```python
from build123d import *

# Parameters (mm, degrees)
F0_W     = 80
F0_H     = 80
F1_DEPTH = 80
F2_R     = 17.5
F3_DEPTH = 25
F4_R     = 17.5
F5_DEPTH = 80.001
F6_T     = -2.5


with BuildPart() as f1:
    # F0 (on Front) → F1 (new body)
    with BuildSketch(Plane.XZ):
        Rectangle(F0_W, F0_H)
    extrude(amount=F1_DEPTH)

    # F2 (on face) → F3 (join)
    with BuildSketch(Plane.XZ.offset(80)):
        Circle(F2_R)
    extrude(amount=F3_DEPTH)

    # F4 (on face) → F5 (cut, through all)
    with BuildSketch(Plane.XY.offset(40)):
        with Locations((0, -40)):
            Circle(F4_R)
    extrude(amount=-F5_DEPTH, mode=Mode.SUBTRACT)

    # F6
    f6_openings = [f1.faces().sort_by_distance(p)[0] for p in [
        (-38.868629, -40, -40),
    ]]
    offset(amount=F6_T, openings=f6_openings, kind=Kind.INTERSECTION)


solid = f1.part
```
Design review of the part built by this model. Coordinates are the model's own, in mm. A direction names the side the tool comes from. Give positions to 0.01 mm unless a question says otherwise; leave off trailing zeros. Order: outer loops, then holes, each group sorted by start corner. A loop starts at its lowest first (then second) coordinate and runs counter-clockwise, first axis right, second up. Notation, with made-up numbers: M 8.25,74.5 L 60.25,74.5 A14 ccw 60.25,82.5 Z; hole C 19.25,43.5 d11. An arc over 180 degrees is marked long. One line per question, with ' | ' between items. Start each with the question number.
Q1. For L1, parallel to Y at x = 0, z = -7; L2, parallel to Y at x = 0, z = 18.5; L3, parallel to Y at x = 35, z = 34.5, list the stretches that pass through material, from the lowest coordinate up. Write a range as [from, to].
Q2. Machinability: for faces 5 (the face through (-37.5, -39, -2)), 6 (the face through (-1, -80, 18)), 7 (the face through (-14.985, -89.825, 0.66)), 8 (the face through (-40, -39, -1)), which of the approach directions +Z, -Z, +X, -X, +Y, -Y give a long, thin tool a straight path to every point of the face, cutting with its end or side? Answer none if there is none.
Q3. We need section D-D (z = 0). Write out the cut boundary in (x, y).
Q4. We need section C-C (y = -40). Write out the cut boundary in (x, z), plus the area to 4 significant figures.
Q5. For pin 1 Ø10 at (x, y) = (20, -87.5) entering from -Z; pin 2 Ø3 at (y, z) = (-94, 14) entering from -X; pin 3 Ø4 at (y, z) = (-82.5, 21) entering from -X; pin 4 Ø2 at (x, z) = (-21.5, -24) entering from -Y, all flat-tipped, find the tip position at first contact; note any pin that passes through.
Q6. The part is to be moulded in two halves that separate along Z. For faces 1 (the face through (-1, -22, 40)), 2 (the face through (40, -39, -1)), 3 (the face through (0, -102.5, 0)), 4 (the face through (-17, -23, 37.5)), say which applies: +Z half, -Z half, draft (parallel to the pull), parting line (faces both ways), or undercut.
Q7. We need section A-A (z = -24). Write out the cut boundary in (x, y).
Q8. We need section B-B (x = 0). Write out the cut boundary in (y, z).
Returned:
1) L1: [-105, -102.5], [-60, -57.5], [-22.5, -20], [-2.5, 0] | L2: [-80, -77.5], [-60, -57.5], [-22.5, -20], [-2.5, 0] | L3: [-80, -77.5], [-2.5, 0]
2) face 5: -Z | face 6: -Y | face 7: none | face 8: +Z, -Z, -X, +Y, -Y
3) outline: M -40,-80 L -17.5,-80 L -17.5,-105 L 17.5,-105 L 17.5,-80 L 40,-80 L 40,0 L -40,0 Z; C 0,-40 d40; hole M -37.5,-77.5 L -15,-77.5 L -15,-102.5 L 15,-102.5 L 15,-77.5 L 37.5,-77.5 L 37.5,-2.5 L -37.5,-2.5 Z; hole C 0,-40 d35
4) outline: M -40,-40 L -37.5,-40 L -37.5,37.5 L -20,37.5 L -20,-40 L -17.5,-40 L -17.5,40 L -40,40 Z; M 17.5,-40 L 20,-40 L 20,37.5 L 37.5,37.5 L 37.5,-40 L 40,-40 L 40,40 L 17.5,40 Z | area: 887.5 mm2
5) pin 1: z = -9.01 | pin 2: x = -12.25 | pin 3: through | pin 4: y = -80
6) face 1: +Z half | face 2: draft | face 3: undercut | face 4: -Z half
7) outline: M -40,-80 L 40,-80 L 40,0 L -40,0 Z; C 0,-40 d40; hole M -37.5,-77.5 L 37.5,-77.5 L 37.5,-2.5 L -37.5,-2.5 Z; hole C 0,-40 d35
8) outline: M -105,-17.5 L -80,-17.5 L -80,-40 L -77.5,-40 L -77.5,-15 L -102.5,-15 L -102.5,15 L -77.5,15 L -77.5,37.5 L -60,37.5 L -60,-40 L -57.5,-40 L -57.5,40 L -80,40 L -80,17.5 L -105,17.5 Z; M -22.5,-40 L -20,-40 L -20,37.5 L -2.5,37.5 L -2.5,-40 L 0,-40 L 0,40 L -22.5,40 Z
